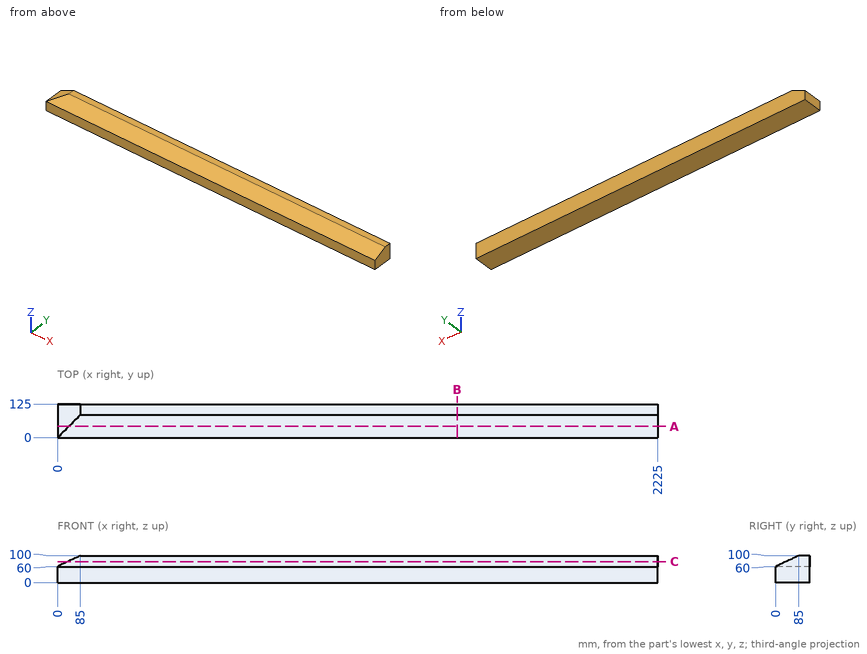
Verification items for this drawing (mm, ordinates from the low corner). Coordinates: 2 decimals unless noted, no trailing zeros. Order: outer loops, then holes, each group sorted by start corner. A loop starts at its lowest first (then second) coordinate and runs counter-clockwise, first axis right, second up. Notation, with made-up numbers: (68, 39.25) -> (78, 39.25) arc R26 ccw to (78, 59.25) -> close; hole circle Ø7 at (42, 1). An arc over 180 degrees is marked (long way). Answer as CSV lines item,"result". Start each with the question number.
1) Gauge pin test, flat ends, axial feed: pin 1 Ø8 at (x, y) = (633, 70) entering from +Z; pin 2 Ø6 at (x, z) = (1281, 68.5) entering from -Y; pin 3 Ø8 at (x, y) = (1749, 73) entering from +Z. Record the tip position at first contact, or that the pin passes through.
2) Cross-section at C-C, the plane z = 78. Record the boundary of the cut face in (x, y).
3) Material ranges on L1, parallel to Z at x = 987.5, y = 47; L2, parallel to Y at x = 223, z = 69.5; L3, parallel to Y at x = 357.5, z = 65.5, recorded low to high. Write a range as [from, to].
4) Cross-section at B-B, the plane x = 1481.5. Record the boundary of the cut face in (y, z).
5) Cross-section at A-A, the plane y = 42.5. Record the boundary of the cut face in (x, z), then the cut area to 3 significant figures.
Conclusion:
1,pin 1,"stops at z = 94.82"
1,pin 2,"stops at y = 11.69"
1,pin 3,"stops at z = 96.24"
2,outline,"(38.25, 38.25) -> (2225, 38.25) -> (2225, 125) -> (38.25, 125) -> close"
3,L1,"z = [0, 82.12]"
3,L2,"y = [20.19, 125]"
3,L3,"y = [11.69, 125]"
4,outline,"(0, 0) -> (125, 0) -> (125, 100) -> (85, 100) -> (0, 60) -> close"
5,outline,"(0, 0) -> (2225, 0) -> (2225, 80) -> (42.5, 80) -> (0, 60) -> close"
5,area,"178,000 mm²"
